Autodesk Inventor part; units mm, degrees
ref_plane "YZ Plane" through (0, 0, 0) normal (1, 0, 0) x (0, 1, 0)
ref_plane "XZ Plane" through (0, 0, 0) normal (0, 1, 0) x (-1, 0, 0)
ref_plane "XY Plane" through (0, 0, 0) normal (0, 0, 1) x (1, 0, 0)
sketch "Sketch1" plane through (0, 0, 0) normal (0, 1, 0) x (-1, 0, 0)
  line L0 (1, 9) -> (-1, 9)
  line L1 (-1, 9) -> (-1, -9)
  line L2 (-1, -9) -> (1, -9)
  line L3 (1, -9) -> (1, 9)
  line L4 (1, 9) -> (-1, -9) construction
  line L5 (-1, 9) -> (1, -9) construction
  line L6 (3.5, -5.5) -> (-3.5, -5.5)
  line L7 (-3.5, -5.5) -> (-3.5, -9)
  line L8 (-3.5, -9) -> (3.5, -9)
  line L9 (3.5, -9) -> (3.5, -5.5)
  line L10 (0, 0) -> (0, -9)
  dimension "d0" = 2
  dimension "d2" = 18
  dimension "d3" = 7
  dimension "d4" = 3.5
extrude "Inserted Base" add sketch "Sketch1" along normal blind 8
sketch "Sketch2" plane through (0, 8, 0) normal (0, 1, 0) x (1, 0, 0)
  line L0 (3.5, 5.5) -> (3.5, 9)
  line L1 (1, 5.5) -> (3.5, 9)
  line L2 (1, 5.5) -> (3.5, 5.5)
  line L3 (3.5, 9) -> (3.5, 5.5)
  line L4 (3.5, 5.5) -> (1, 5.5)
  line L5 (-1, 5.5) -> (-3.5, 9)
  line L6 (-3.5, 9) -> (-3.5, 5.5)
  line L7 (-3.5, 9) -> (-3.5, 5.5)
  line L8 (-3.5, 5.5) -> (-1, 5.5)
  line L9 (-3.5, 5.5) -> (-1, 5.5)
  point P0 (0, 0)
extrude "Triangle Edges" cut sketch "Sketch2" against normal through all
sketch "Sketch3" plane through (0, 8, 0) normal (0, 1, 0) x (1, 0, 0)
  line L0 (-1, -9) -> (1, -9)
  line L1 (1, -9) -> (1, -41.5)
  line L2 (1, -41.5) -> (-1, -41.5)
  line L3 (-1, -41.5) -> (-1, -9)
  line L4 (1, -9) -> (1, 5.5)
  line L5 (-1, -39.5) -> (1, -39.5)
  line L6 (-1, 5.5) -> (-1, -9)
  line L7 (1, 5.5) -> (-1, 5.5)
  point P0 (0, 0)
  dimension "d9" = 2
  dimension "d14" = 45
extrude "Tab Extension" add sketch "Sketch3" against normal blind 6 contours L0 L1 L5 L3 | L5 L1 L2 L3
sketch "Sketch4" plane through (0, 8, 0) normal (0, 1, 0) x (1, 0, 0)
  line L0 (2, -39.5) -> (-2, -39.5)
  line L1 (-2, -39.5) -> (-2, -37.5)
  line L2 (-2, -37.5) -> (2, -37.5)
  line L3 (2, -37.5) -> (2, -39.5)
  line L4 (1, -9) -> (1, 5.5)
  line L5 (-1, 5.5) -> (-1, -9)
  line L6 (1, 5.5) -> (-1, 5.5)
  line L7 (0, 0) -> (0, 5.5)
  line L8 (-1, -41.5) -> (-1, -9)
  dimension "d13" = 45
  dimension "d15" = 2
  dimension "d16" = 1
extrude "Electrode rest" add sketch "Sketch4" against normal up to surface (6 mm away)
sketch "Sketch5" plane through (0, 8, 0) normal (0, 1, 0) x (1, 0, 0)
  line L0 (-1, -34.5) -> (1, -34.5)
  line L1 (1, -9) -> (1, -37.5)
  line L2 (-2, -37.5) -> (-1, -37.5)
  line L3 (-2, -37.5) -> (-1, -37.5)
  line L4 (-1, -34.5) -> (-2, -37.5)
  line L5 (2, -37.5) -> (1, -37.5)
  line L6 (1, -37.5) -> (2, -37.5)
  line L7 (2, -37.5) -> (1, -34.5)
  line L8 (-1, -37.5) -> (-1, -34.5)
  line L9 (-1, -37.5) -> (-1, -9)
  point P0 (0, 0)
  dimension "d19" = 3
extrude "Taper" add sketch "Sketch5" against normal up to surface (6 mm away)
properties part number "tabwtip_2mm_1128"
Here's how the part is built. I have some questions about the finished solid (model axes, mm). A direction names the side the tool comes from. Give positions to 0.01 mm unless a question says otherwise; leave off trailing zeros. Loops run counter-clockwise (first coordinate to the right, second up) from the corner with the lowest first, then second, coordinate; pieces in that order, holes last. Notation, with made-up numbers: M 52.25,34.25 L 84.25,34.25 A24 ccw 84.25,72.25 Z; hole C 69.5,13.5 d10. An arc over 180 degrees is marked long. Put each result on its own line as item: value. Start each with the question number.
(1) I need wall thicknesses on line 1 along Y through (x, z) = (-0.75, 24); line 2 along X through (y, z) = (2.5, 4); line 3 along Z through (x, y) = (-1.25, 0.5). Which ranges of each line are inside material? Lowest first, please. Write a range as [from, to].
(2) I want a section at B-B on x = 0.5. Please give me the cut outline in (y, z), then the cut area to 3 significant figures.
(3) Will these pins go through, and if not, where does the flat tip stop? pin 1 Ø1 at (x, y) = (-2, 2.5) entering from +Z; pin 2 Ø2.5 at (y, z) = (3.5, 7.5) entering from +X; pin 3 Ø3 at (x, z) = (0.5, 24.5) entering from -Y; pin 4 Ø4 at (x, y) = (1.5, 3) entering from +Z.
(4) I want a section at C-C on z = 20. Please give me the cut outline in (x, y).
(5) I want a section at D-D on y = 1. Please give me the cut outline in (x, z).
(6) I want a section at A-A on y = 4.5. Please give me the cut outline in (x, z).
(7) If we mould it in two halves opening along Z, with no side actions, what happens to faces 1 (the flat face through (0, 2, 25)), 2 (the flat face through (1, 5, 15)), 3 (the flat face through (-1.5, 5, 39.5)), 4 (the flat face through (1.5, 5, 36))? For each: +Z half, -Z half, draft (parallel to the pull), parting line (faces both ways), or undercut.
(8) For faces 5 (the flat face through (-1.5, 5, 36)), 6 (the flat face through (-2, 5, 39)), 7 (the flat face through (2.233, 4.056, -7.225)), which set-ups out of +Z, -Z, +X, -X, +Y, -Y let a thin tool reach every point of the face, with its end or its side?
Answer block:
1. line 1: [2, 8]
1. line 2: [-1, 1]
1. line 3: [-9, -5.85]
2. outline: M 0,-9 L 8,-9 L 8,41.5 L 2,41.5 L 2,9 L 0,9 Z
2. area: 339 mm^2
3. pin 1: z = 39.5
3. pin 2: x = 1
3. pin 3: y = 2
3. pin 4: z = 41.5
4. outline: M -1,2 L 1,2 L 1,8 L -1,8 Z
5. outline: M -3.5,-9 L 3.5,-9 L 1,-5.5 L 1,9 L -1,9 L -1,-5.5 Z
6. outline: M -3.5,-9 L 3.5,-9 L 1,-5.5 L 1,34.5 L 2,37.5 L 2,39.5 L 1,39.5 L 1,41.5 L -1,41.5 L -1,39.5 L -2,39.5 L -2,37.5 L -1,34.5 L -1,-5.5 Z
7. face 1: draft
7. face 2: undercut
7. face 3: +Z half
7. face 4: undercut
8. face 5: -X, +Y, -Y
8. face 6: +Z, -X, +Y, -Y
8. face 7: +X, +Y, -Y
